Read the model definition and answer for the solid it produces. Units are mm, in the model's axes. A direction names the side the tool comes from. Coordinates: 2 decimals unless noted, no trailing zeros. Order: outer loops, then holes, each group sorted by start corner. A loop starts at its lowest first (then second) coordinate and runs counter-clockwise, first axis right, second up. Notation, with made-up numbers: M 12.25,32 L 63.25,32 A11 cw 63.25,40 Z; hole C 5,26 d11. An arc over 180 degrees is marked long. Use a Markdown table: item, result. Add a question column.
1) Find the intervals of material crossed by probe 1 along Y at (x, z) = (-40.5, 9.5); probe 2 along Y at (x, z) = (-31.75, 2.25); probe 3 along Y at (x, z) = (-38.25, 2), in increasing order. Write a range as [from, to].
2) Find section B-B on y = 23.75. Write down the section's boundary in (x, z), plus the area to 3 significant figures.
3) Find section C-C on x = -35.5. Write down the section's boundary in (y, z).
4) Find section D-D on x = -33.5. Write down the section's boundary in (y, z).
5) The mould has two halves that part along Y. Classify faces 1 (the face through (-36, 28, 0)), 2 (the face through (-36, 28, 4)), 3 (the face through (-36, 38.038, 5)), 4 (the face through (-36, 25, 9)): released by +Y, released by -Y, zero draft, split by the parting line, or undercut.
6) Find section A-A on z = 6.25. Write down the section's boundary in (x, y), plus the area to 3 significant figures.
7) For faces 5 (the face through (-44.459, 28.1, 3.8)), 6 (the face through (-36, 31, 8)), determine the directions among +Z, -Z, +X, -X, +Y, -Y from which every point of the face is accessible in a straight line to the end or side of a thin tool.
Solid Edge part; units mm, degrees
sketch "Sketch1" plane through (0, 0, 0) normal (0, 0, 1) x (1, 0, 0)
  circle A0 centre (-32.934, 22.9674) radius 1.7
  line L0 (-44.4588, 17.9674) -> (-27.934, 17.9674)
  line L1 (-27.934, 17.9674) -> (-27.934, 38.0385)
  line L2 (-27.934, 38.0385) -> (-44.4588, 38.0385)
  line L3 (-44.4588, 38.0385) -> (-44.4588, 17.9674)
  circle A1 centre (-39.4588, 33.0385) radius 1.7
  dimension "D1" = 39.4588
  dimension "D2" = 32.934
extrude "Protrusion1" add sketch "Sketch1" along normal blind 10
sketch "Sketch2" plane through (-44.4588, 28.0029, 5) normal (-1, 0, 0) x (0, -1, 0)
  line L0 (-2.9971, 2) -> (-2.9971, 7.3405)
  line L1 (-2.9971, 7.3405) -> (3.0029, 7.3405)
  line L2 (3.0029, 7.3405) -> (3.0029, 2)
  arc A0 (3.0029, 2) -> (-2.9971, 2) centre (0.0029, 2) cw
extrude "Cutout1" cut sketch "Sketch2" against normal through all
Check result:
| question | item | result |
|---|---|---|
| 1 | probe 1 | y = [17.97, 25], [31, 31.69], [34.38, 38.04] |
| 1 | probe 2 | y = [17.97, 21.75], [24.19, 38.04] |
| 1 | probe 3 | y = [17.97, 31.84], [34.23, 38.04] |
| 2 | outline | M -44.46,0 L -34.44,0 L -34.44,10 L -44.46,10 Z; M -31.42,0 L -27.93,0 L -27.93,10 L -31.42,10 Z |
| 2 | area | 135 mm2 |
| 3 | outline | M 17.97,0 L 38.04,0 L 38.04,10 L 31,10 L 31,7 A3 cw 25,7 L 25,10 L 17.97,10 Z |
| 4 | outline | M 17.97,0 L 21.36,0 L 21.36,10 L 17.97,10 Z; M 24.57,0 L 38.04,0 L 38.04,10 L 31,10 L 31,7 A3 cw 25,7 L 25,10 L 24.57,10 Z |
| 5 | face 1 | zero draft |
| 5 | face 2 | undercut |
| 5 | face 3 | released by +Y |
| 5 | face 4 | undercut |
| 6 | outline | M -44.46,17.97 L -27.93,17.97 L -27.93,25.1 L -44.46,25.1 Z; M -44.46,30.9 L -27.93,30.9 L -27.93,38.04 L -44.46,38.04 Z; hole C -39.46,33.04 d3.4; hole C -32.93,22.97 d3.4 |
| 6 | area | 218 mm2 |
| 7 | face 5 | +Z, -Z, -X, +Y, -Y |
| 7 | face 6 | +Z, +X, -X |
